```python
from build123d import *

# Parameters (mm, degrees)
F0_R     = 2
F1_DEPTH = 5


with BuildPart() as f1:
    # F0 (on Top) → F1 (new body)
    with BuildSketch(Plane.XY):
        with BuildLine():
            ThreePointArc((-1.8593732966, 3.5415718183), (0.1256674698, 3.9980254735), (2.0781231578, 3.4178069198))
            Line((2.0781231578, 3.4178069198), (2.0781231578, 9.95312538))
            Line((2.0781231578, 9.95312538), (-1.8593732966, 13.2343750447))
            Line((-1.8593732966, 13.2343750447), (-1.8593732966, 3.5415718183))
        make_face()
        with BuildLine():
            ThreePointArc((3.3147150847, -2.2388979224), (3.8248438098, -1.1707133853), (4, 0))
            ThreePointArc((4, 0), (3.4865808919, 1.9605493323), (2.0781231578, 3.4178069198))
            ThreePointArc((2.0781231578, 3.4178069198), (0.1256674698, 3.9980254735), (-1.8593732966, 3.5415718183))
            ThreePointArc((-1.8593732966, 3.5415718183), (-3.9093033939, 0.8469633845), (-3.1584306628, -2.4544481556))
            ThreePointArc((-3.1584306628, -2.4544481556), (0.1331228038, -3.9977841762), (3.3147150847, -2.2388979224))
        make_face()
        Circle(F0_R, mode=Mode.SUBTRACT)
        with BuildLine():
            add(Edge.make_bspline(
                [(3.3147150847, -2.2388979224), (2.7708082025, -7.9966705645), (1.7749881346, -18.5865607153), (-4.9275215468, -23.4735932789), (-7.9843755811, -25.7031265646)],
                knots=[0, 0, 0, 0, 0.5438220711, 1, 1, 1, 1], degree=3))
            ThreePointArc((3.3147150847, -2.2388979224), (0.1331228038, -3.9977841762), (-3.1584306628, -2.4544481556))
            add(Edge.make_bspline(
                [(-3.1584306628, -2.4544481556), (-2.9708882556, -7.7977456433), (-1.9257495096, -17.6899848541), (-6.6804976422, -22.9462452047), (-7.9843755811, -25.7031265646)],
                knots=[0, 0, 0, 0, 0.5577685344, 1, 1, 1, 1], degree=3))
        make_face()
    extrude(amount=F1_DEPTH)


solid = f1.part
```
Part model, mm, in its own coordinate system. A direction names the side the tool comes from. Coordinates: 2 decimals unless noted, no trailing zeros. Order: outer loops, then holes, each group sorted by start corner. A loop starts at its lowest first (then second) coordinate and runs counter-clockwise, first axis right, second up. Notation, with made-up numbers: (30.25, -33.5) - (35.25, -33.5) arc R33 ccw to (35.25, -0.5) - close; hole circle Ø2 at (75.25, -2). An arc over 180 degrees is marked (long way). Return JSON: item names as keys, results as strings. Group by question number.
Item 1: Which spindle directions (+Z, -Z, +X, -X, +Y, -Y) get a long thin tool onto all of the face, cutting with end or side? Do faces 1 (the face through (-1.859, 8, 2)), 2 (the face through (0.1, 11.6, 2.5)). Say none if no direction does.
Item 2: Pull direction X, two halves, no side cores. Call faces 3 (the face through (2.078, 7, 2)), 4 (the face through (0, -2, 2)), 5 (the face through (0, -6, 0)), 6 (the face through (-3.9, 0.89, 2.46)): pulls with the +X half, pulls with the -X half, needs draft (parallel to the pull), parting line crosses it, or undercut.
Item 3: Cut at B-B (y = 6). List the corners of the cut face in (x, z), plus the area to 3 significant figures.
Item 4: Pin check, flat tips, straight feed: pin 1 (2.5 mm diameter, centred on y = 10, z = 2.5, fed in from -X); pin 2 (1 mm diameter, centred on y = 0, z = 1, fed in from -X); pin 3 (1.5 mm diameter, centred on y = -2.5, z = 3, fed in from +X). Stop position of each tip, or through.
Item 5: Drill centre lines: probe 1 along Y at (x, z) = (0, 2.9); probe 2 along X at (y, z) = (-1, 2.05); probe 3 along X at (y, z) = (2.5, 4.05). Where is each one in solid material? Low to high. Write a range as from..to.
Item 6: Cut at A-A (y = -1.5). List the corners of the cut face in (x, z), plus the area to 3 significant figures.
Check values:
{
 "1": {"face 1": "+Z, -Z, -X, +Y", "face 2": "+Z, -Z, +X, +Y"},
 "2": {"face 3": "pulls with the +X half", "face 4": "undercut", "face 5": "needs draft", "face 6": "pulls with the -X half"},
 "3": {"outline": "(-1.86, 0) - (2.08, 0) - (2.08, 5) - (-1.86, 5) - close", "area": "19.7 mm2"},
 "4": {"pin 1": "stops at x = -1.86", "pin 2": "stops at x = -4", "pin 3": "stops at x = 3.6"},
 "5": {"probe 1": "y = -17.83..-2, 2..11.68", "probe 2": "x = -3.87..-1.73, 1.73..3.87", "probe 3": "x = -3.12..3.12"},
 "6": {"outline": "(-3.71, 0) - (-1.32, 0) - (-1.32, 5) - (-3.71, 5) - close; (1.32, 0) - (3.71, 0) - (3.71, 5) - (1.32, 5) - close", "area": "23.9 mm2"}
}
